from build123d import *

# Parameters (mm, degrees)
ESBO_O1_R                  = 7
RESSALTO_EXTRUS_O1_DEPTH   = 60
ESBO_O2_R                  = 6
CORTE_EXTRUS_O1_DEPTH      = 71
CORTE_EXTRUS_O2_DEPTH      = 21
CORTE_EXTRUS_O2_DEPTH_BACK = 21
ESBO_O3_W                  = 6.357761197
ESBO_O3_H                  = 12.7967598


with BuildPart() as part:
    # Esboço1 → Ressalto-extrusão1 (new body)
    with BuildSketch(Plane.XY):
        with Locations((-19.442180611, 6.398692353)):
            Circle(ESBO_O1_R)
    extrude(amount=RESSALTO_EXTRUS_O1_DEPTH)

    # Esboço2 → Corte-extrusão1 (cut)
    with BuildSketch(Plane.XY.offset(60)):
        with Locations((-19.442180611, 6.398692353)):
            Circle(ESBO_O2_R)
    extrude(amount=-CORTE_EXTRUS_O1_DEPTH, mode=Mode.SUBTRACT)

    # Esboço3 → Corte-extrusão2 (cut, two sides: drawn at the far end of the back side and taken through both)
    with BuildSketch(Plane(origin=(0, 0, 0), x_dir=(1, 0, 0), z_dir=(0, 1, 0)).offset(-CORTE_EXTRUS_O2_DEPTH_BACK)):
        with Locations((-19.265634303, -29.9983799)):
            Rectangle(ESBO_O3_W, ESBO_O3_H)
    extrude(amount=CORTE_EXTRUS_O2_DEPTH + CORTE_EXTRUS_O2_DEPTH_BACK, mode=Mode.SUBTRACT)


solid = part.part
For this review, take the finished solid that the model builds, in its own axes (mm). A direction names the side the tool comes from. Give positions to 0.01 mm unless a question says otherwise; leave off trailing zeros. Order: outer loops, then holes, each group sorted by start corner. A loop starts at its lowest first (then second) coordinate and runs counter-clockwise, first axis right, second up. Notation, with made-up numbers: M -36,-16 L 0,-16 A12 cw 0,-6 Z; hole C -39.75,75.5 d10. An arc over 180 degrees is marked long. Answer in a Markdown table with one row per item. Add a question column.
(1) Consider section B-B on y = 7.75. State the section outline as (x, z) points, and give its area (3 significant figures).
(2) Consider section D-D on x = -17.75. State the section outline as (y, z) points.
(3) Consider section C-C on x = -20. State the section outline as (y, z) points.
(4) Consider section A-A on z = 25. State the section outline as (x, y) points, and give its area (3 significant figures).
(5) Wall thickness on probe 1 along Y at (x, z) = (-19.75, 49.5); probe 2 along Z at (x, y) = (-21.5, 13); probe 3 along X at (y, z) = (5.75, 56): over which ranges is each line inside the solid? List them lowest first. Write a range as [from, to].
(6) Mouldability with a two-part tool opening along Z and no side actions: class faces 1 (the face through (-22.445, 1, 30)), 2 (the face through (-14, 10, 0)), 3 (the face through (-14, 10, 60)) as +Z half, -Z half, draft (parallel to the pull), parting line (faces both ways), or undercut.
(7) For pin 1 (0.6 mm diameter, centred on y = 12, z = 31.5, fed in from -X); pin 2 (6 mm diameter, centred on x = -23, z = 31, fed in from -Y); pin 3 (1.5 mm diameter, centred on y = 8.5, z = 41, fed in from -X), all flat-tipped, find the tip position at first contact; note any pin that passes through.
(8) For faces 4 (the face through (-25.436, 6.663, 30.42)), 5 (the face through (-19, 13, 23.6)), list the 3-axis set-ups (+Z, -Z, +X, -X, +Y, -Y) from which the entire face can be reached by the end or side of a thin tool; tool diameter is ignored.
Evaluation:
| question | item | result |
|---|---|---|
| 1 | outline | M -26.31,0 L -25.29,0 L -25.29,60 L -26.31,60 Z; M -13.6,0 L -12.57,0 L -12.57,60 L -13.6,60 Z |
| 1 | area | 123 mm^2 |
| 2 | outline | M -0.39,0 L 0.64,0 L 0.64,23.6 L -0.39,23.6 Z; M -0.39,36.4 L 0.64,36.4 L 0.64,60 L -0.39,60 Z; M 12.16,0 L 13.19,0 L 13.19,23.6 L 12.16,23.6 Z; M 12.16,36.4 L 13.19,36.4 L 13.19,60 L 12.16,60 Z |
| 3 | outline | M -0.58,0 L 0.42,0 L 0.42,23.6 L -0.58,23.6 Z; M -0.58,36.4 L 0.42,36.4 L 0.42,60 L -0.58,60 Z; M 12.37,0 L 13.38,0 L 13.38,23.6 L 12.37,23.6 Z; M 12.37,36.4 L 13.38,36.4 L 13.38,60 L 12.37,60 Z |
| 4 | outline | M -22.44,0.08 L -22.44,1.2 A6 cw -22.44,11.59 L -22.44,12.72 A7 ccw Z; M -16.09,0.26 A7 ccw -16.09,12.54 L -16.09,11.37 A6 cw -16.09,1.42 Z |
| 4 | area | 27.5 mm^2 |
| 5 | probe 1 | y = [-0.59, 0.41], [12.39, 13.39] |
| 5 | probe 2 | z = [0, 23.6], [36.4, 60] |
| 5 | probe 3 | x = [-26.41, -25.41], [-13.48, -12.47] |
| 6 | face 1 | undercut |
| 6 | face 2 | -Z half |
| 6 | face 3 | +Z half |
| 7 | pin 1 | stops at x = -24.01 |
| 7 | pin 2 | stops at y = 0.08 |
| 7 | pin 3 | stops at x = -26.31 |
| 8 | face 4 | +Z, -Z |
| 8 | face 5 | +Y, -Y |
